from build123d import *

# Parameters (mm, degrees)
ESBO_O1_W                  = 58
ESBO_O1_H                  = 24.5
RESSALTO_EXTRUS_O1_DEPTH   = 107.92
FILETE1_R                  = 5
ESBO_O2_W                  = 44
ESBO_O2_H                  = 93.92
CORTE_EXTRUS_O1_DEPTH      = 19
FILETE2_R                  = 5
ESBO_O3_R                  = 3.5
CORTE_EXTRUS_O2_DEPTH      = 20
CORTE_EXTRUS_O2_DEPTH_BACK = 6.5


with BuildPart() as part:
    # Esboço1 → Ressalto-extrusão1 (new body)
    with BuildSketch(Plane(origin=(0, 0, 0), x_dir=(1, 0, 0), z_dir=(0, 1, 0))):
        Rectangle(ESBO_O1_W, ESBO_O1_H)
    extrude(amount=RESSALTO_EXTRUS_O1_DEPTH)

    # Filete1
    filete1_edges = [part.edges().sort_by_distance(p)[0] for p in [
        (29, 107.92, 0),
        (-29, 107.92, 0),
        (29, 0, 0),
        (-29, 0, 0),
    ]]
    fillet(filete1_edges, radius=FILETE1_R)

    # Esboço2 → Corte-extrusão1 (cut)
    with BuildSketch(Plane.XY.offset(12.25)):
        with Locations((0, 53.96)):
            Rectangle(ESBO_O2_W, ESBO_O2_H)
    extrude(amount=-CORTE_EXTRUS_O1_DEPTH, mode=Mode.SUBTRACT)

    # Filete2
    filete2_edges = [part.edges().sort_by_distance(p)[0] for p in [
        (-22, 7, 2.75),
        (-22, 100.92, 2.75),
        (22, 100.92, 2.75),
        (22, 7, 2.75),
    ]]
    fillet(filete2_edges, radius=FILETE2_R)

    # Esboço3 → Corte-extrusão2 (cut, two sides)
    with BuildSketch(Plane.XY.offset(-6.75)) as corte_extrus_o2_sk:
        with Locations((0, 79.92)):
            Circle(ESBO_O3_R)
        with Locations((0, 45.4387)):
            Circle(ESBO_O3_R)
    extrude(amount=CORTE_EXTRUS_O2_DEPTH, mode=Mode.SUBTRACT)
    extrude(corte_extrus_o2_sk.sketch, amount=-CORTE_EXTRUS_O2_DEPTH_BACK, mode=Mode.SUBTRACT)


solid = part.part
Work out the finished part from the listing and answer in its coordinate system (mm). A direction names the side the tool comes from. Round coordinates to 2 decimals unless told otherwise and drop trailing zeros. Write each loop counter-clockwise with the first axis right and the second up, starting at its lowest first coordinate (ties: lowest second). Pieces come first, ordered by that corner, then holes.
1) A cutting plane is placed at A-A (x = 0). Give the vertices of the cut face in (y, z).
2) A tool of negligible diameter and unlimited length cuts with its end or side. For faces 4 (the cylindrical face through (-20.57, 99.42, 2.62)), 5 (the flat face through (-26, 53, 12.25)), from which of +Z, -Z, +X, -X, +Y, -Y can it reach the whole face along a straight path? Write none if from no direction.
3) A cutting plane is placed at B-B (y = 79.92). Give the vertices of the cut face in (x, z).
4) Given pin 1 Ø13 at (x, y) = (4.5, 70) entering from +Z; pin 2 Ø4 at (x, y) = (0, 45.44) entering from -Z, each flat-ended and moving along its own axis, determine where each tip first touches the part or whether it passes through.
5) The mould has two halves that part along X. Classify faces 1 (the flat face through (0, 100.92, 3)), 2 (the flat face through (0, 107.92, 0)), 3 (the cylindrical face through (-28, 2, 0)): pulls with the +X half, pulls with the -X half, needs draft (parallel to the pull), parting line crosses it, or undercut.
6) A cutting plane is placed at D-D (y = 23.5). Give the vertices of the cut face in (x, z).
7) Straight lines are drawn through the part: line 1 (Y direction, x = 0, z = -8.6); line 2 (Y direction, x = -13.5, z = 3.5); line 3 (X direction, y = 77, z = 1). For each, find the intervals that lie inside material, in ascending order.
8) A cutting plane is placed at C-C (z = 7.5). Give the vertices of the cut face in (x, y), plus the area to 3 significant figures.
Completed:
1. outline: (0, -12.25) - (41.94, -12.25) - (41.94, -6.75) - (7, -6.75) - (7, 12.25) - (0, 12.25) - close; (48.94, -12.25) - (76.42, -12.25) - (76.42, -6.75) - (48.94, -6.75) - close; (83.42, -12.25) - (107.92, -12.25) - (107.92, 12.25) - (100.92, 12.25) - (100.92, -6.75) - (83.42, -6.75) - close
2. face 4: +Z
2. face 5: +Z, +X, -X, +Y, -Y
3. outline: (-29, -12.25) - (-3.5, -12.25) - (-3.5, -6.75) - (-22, -6.75) - (-22, 12.25) - (-29, 12.25) - close; (3.5, -12.25) - (29, -12.25) - (29, 12.25) - (22, 12.25) - (22, -6.75) - (3.5, -6.75) - close
4. pin 1: stops at z = -6.75
4. pin 2: passes through
5. face 1: undercut
5. face 2: needs draft
5. face 3: pulls with the -X half
6. outline: (-29, -12.25) - (29, -12.25) - (29, 12.25) - (22, 12.25) - (22, -6.75) - (-22, -6.75) - (-22, 12.25) - (-29, 12.25) - close
7. line 1: y = 0 to 41.94, 48.94 to 76.42, 83.42 to 107.92
7. line 2: y = 0 to 7, 100.92 to 107.92
7. line 3: x = -29 to -22, 22 to 29
8. outline: (-29, 5) arc R5 ccw to (-24, 0) - (24, 0) arc R5 ccw to (29, 5) - (29, 102.92) arc R5 ccw to (24, 107.92) - (-24, 107.92) arc R5 ccw to (-29, 102.92) - close; hole (-22, 12) arc R5 ccw to (-17, 7) - (17, 7) arc R5 ccw to (22, 12) - (22, 95.92) arc R5 ccw to (17, 100.92) - (-17, 100.92) arc R5 ccw to (-22, 95.92) - close
8. area: 2,130 mm2
